```python
from build123d import *

# Parameters (mm, degrees)
SKETCH1_W           = 10
SKETCH1_H           = 12.5
SKETCH1_W_2         = 91
SKETCH1_H_2         = 10
SKETCH1_R           = 1.75
BOSS_EXTRUDE1_DEPTH = 3
SKETCH1_3_W         = 2
SKETCH1_3_H         = 10
SKETCH1_3_W_2       = 10
SKETCH1_3_H_2       = 2
BOSS_EXTRUDE2_DEPTH = 24
SKETCH2_W           = 10
SKETCH2_H           = 5
SKETCH2_W_2         = 5
SKETCH2_H_2         = 10
BOSS_EXTRUDE3_DEPTH = 2
SKETCH3_R           = 1.75
CUT_EXTRUDE1_DEPTH  = 12


with BuildPart() as part:
    # Sketch1 → Boss-Extrude1 (new body)
    # profile 1 of 5: a face of its own
    with BuildSketch(Plane(origin=(0, 0, 0), x_dir=(1, 0, 0), z_dir=(0, 1, 0))):
        with Locations((-10.142857143, 23.178571429)):
            Rectangle(SKETCH1_W, SKETCH1_H)
    # profile 2 of 5: a face of its own
    with BuildSketch(Plane(origin=(0, 0, 0), x_dir=(1, 0, 0), z_dir=(0, 1, 0))):
        with Locations((10.357142857, 11.928571429)):
            Rectangle(SKETCH1_W_2, SKETCH1_H_2)
        with Locations(Location((30.357142857, 11.928571429, 0), (0, 0, 270))):
            Circle(SKETCH1_R, mode=Mode.SUBTRACT)
        with Locations(Location((-9.642857143, 11.928571429, 0), (0, 0, 270))):
            Circle(SKETCH1_R, mode=Mode.SUBTRACT)
    # profile 3 of 5: a face of its own
    with BuildSketch(Plane(origin=(0, 0, 0), x_dir=(1, 0, 0), z_dir=(0, 1, 0))):
        with Locations((-10.142857143, 0.678571429)):
            Rectangle(SKETCH1_W, SKETCH1_H)
    # profile 4 of 5: a face of its own
    with BuildSketch(Plane(origin=(0, 0, 0), x_dir=(1, 0, 0), z_dir=(0, 1, 0))):
        with Locations((30.857142857, 0.678571429)):
            Rectangle(SKETCH1_W, SKETCH1_H)
    # profile 5 of 5: a face of its own
    with BuildSketch(Plane(origin=(0, 0, 0), x_dir=(1, 0, 0), z_dir=(0, 1, 0))):
        with Locations((30.857142857, 23.178571429)):
            Rectangle(SKETCH1_W, SKETCH1_H)
    extrude(amount=BOSS_EXTRUDE1_DEPTH)

    # Sketch1_3 → Boss-Extrude2 (add)
    with BuildSketch(Plane(origin=(0, 0, 0), x_dir=(1, 0, 0), z_dir=(0, 1, 0))):
        with Locations((-36.142857143, 11.928571429)):
            Rectangle(SKETCH1_3_W, SKETCH1_3_H)
        with Locations((-10.142857143, -6.571428571)):
            Rectangle(SKETCH1_3_W_2, SKETCH1_3_H_2)
        with Locations((30.857142857, -6.571428571)):
            Rectangle(SKETCH1_3_W_2, SKETCH1_3_H_2)
        with Locations((56.857142857, 11.928571429)):
            Rectangle(SKETCH1_3_W, SKETCH1_3_H)
        with Locations((30.857142857, 30.428571429)):
            Rectangle(SKETCH1_3_W_2, SKETCH1_3_H_2)
        with Locations((-10.142857143, 30.428571429)):
            Rectangle(SKETCH1_3_W_2, SKETCH1_3_H_2)
    extrude(amount=BOSS_EXTRUDE2_DEPTH)

    # Sketch2 → Boss-Extrude3 (add)
    with BuildSketch(Plane(origin=(0, 24, 0), x_dir=(1, 0, 0), z_dir=(0, 1, 0))):
        with Locations((-10.142857143, 28.928571429)):
            Rectangle(SKETCH2_W, SKETCH2_H)
        with Locations((30.857142857, 28.928571429)):
            Rectangle(SKETCH2_W, SKETCH2_H)
        with Locations((55.357142857, 11.928571429)):
            Rectangle(SKETCH2_W_2, SKETCH2_H_2)
        with Locations((30.857142857, -5.071428571)):
            Rectangle(SKETCH2_W, SKETCH2_H)
        with Locations((-10.142857143, -5.071428571)):
            Rectangle(SKETCH2_W, SKETCH2_H)
        with Locations((-34.642857143, 11.928571429)):
            Rectangle(SKETCH2_W_2, SKETCH2_H_2)
    extrude(amount=BOSS_EXTRUDE3_DEPTH)

    # Sketch3 → Cut-Extrude1 (cut)
    with BuildSketch(Plane.XZ):
        with Locations(Location((-10.142857143, -25.428571429, 0), (0, 0, 270))):
            Circle(SKETCH3_R)
        with Locations(Location((30.857142857, -25.428571429, 0), (0, 0, 270))):
            Circle(SKETCH3_R)
    extrude(amount=-CUT_EXTRUDE1_DEPTH, mode=Mode.SUBTRACT)


solid = part.part
```
Geometry: final body of the model. Coordinates: model frame, mm. A direction names the side the tool comes from. Round coordinates to 2 decimals unless told otherwise and drop trailing zeros. Order: outer loops, then holes, each group sorted by start corner. A loop starts at its lowest first (then second) coordinate and runs counter-clockwise, first axis right, second up. Notation, with made-up numbers: (19.25, 44.25) -> (34.25, 44.25) arc R37 ccw to (34.25, 80.25) -> close; hole circle Ø8 at (52, -36). An arc over 180 degrees is marked (long way). Use one line per item in the form item = value.
(1) Section D-D on z = -11.5. Return loops of the section in (x, y), and give its area (3 significant figures).
Results list:
outline = (-37.14, 0) -> (-11.34, 0) -> (-11.34, 3) -> (-35.14, 3) -> (-35.14, 24) -> (-32.14, 24) -> (-32.14, 26) -> (-37.14, 26) -> close; (-7.95, 0) -> (28.66, 0) -> (28.66, 3) -> (-7.95, 3) -> close; (32.05, 0) -> (57.86, 0) -> (57.86, 26) -> (52.86, 26) -> (52.86, 24) -> (55.86, 24) -> (55.86, 3) -> (32.05, 3) -> close
area = 369 mm^2
(2) Section B-B on z = 4. Return loops of the section in (x, y), and give its area (3 significant figures).
Results list:
outline = (-15.14, 0) -> (-5.14, 0) -> (-5.14, 3) -> (-15.14, 3) -> close; (-15.14, 24) -> (-5.14, 24) -> (-5.14, 26) -> (-15.14, 26) -> close; (25.86, 0) -> (35.86, 0) -> (35.86, 3) -> (25.86, 3) -> close; (25.86, 24) -> (35.86, 24) -> (35.86, 26) -> (25.86, 26) -> close
area = 100 mm^2
(3) Draft query along Y for faces 1 (the face through (-10, 13, -29.429)), 2 (the face through (-10, 26, 5)), 3 (the face through (31, 25, -26.429)). Return one class per face: pulls with the +Y half, pulls with the -Y half, needs draft (parallel to the pull), parting line crosses it, or undercut.
Results list:
face_1 = undercut
face_2 = pulls with the +Y half
face_3 = needs draft
(4) Section A-A on y = 8. Return loops of the section in (x, z), and give its area (3 significant figures).
Results list:
outline = (-37.14, -16.93) -> (-35.14, -16.93) -> (-35.14, -6.93) -> (-37.14, -6.93) -> close; (-15.14, -31.43) -> (-5.14, -31.43) -> (-5.14, -29.43) -> (-15.14, -29.43) -> close; (-15.14, 5.57) -> (-5.14, 5.57) -> (-5.14, 7.57) -> (-15.14, 7.57) -> close; (25.86, -31.43) -> (35.86, -31.43) -> (35.86, -29.43) -> (25.86, -29.43) -> close; (25.86, 5.57) -> (35.86, 5.57) -> (35.86, 7.57) -> (25.86, 7.57) -> close; (55.86, -16.93) -> (57.86, -16.93) -> (57.86, -6.93) -> (55.86, -6.93) -> close
area = 120 mm^2
(5) Section C-C on x = -7. Return loops of the section in (y, z).
Results list:
outline = (0, -31.43) -> (26, -31.43) -> (26, -26.43) -> (24, -26.43) -> (24, -29.43) -> (3, -29.43) -> (3, 5.57) -> (24, 5.57) -> (24, 2.57) -> (26, 2.57) -> (26, 7.57) -> (0, 7.57) -> close
(6) Ray query, probe 1 along X at (y, z) = (20.5, -16.5); probe 2 along X at (y, z) = (25, 4.5); probe 3 along Y at (x, z) = (53.5, -7). Return the intervals inside material, ascending. Write a range as [from, to].
Results list:
probe_1 = [-37.14, -35.14], [55.86, 57.86]
probe_2 = [-15.14, -5.14], [25.86, 35.86]
probe_3 = [0, 3], [24, 26]
(7) Access query for faces 4 (the face through (54, 24, -12)), 5 (the face through (31, 25, 2.571)), 6 (the face through (52.857, 25, -12)). Directions: +Z, -Z, +X, -X, +Y, -Y. A direction counts if a zero-diameter tool reaches every point of the face in a straight line with its end or side. Return the directions, or none.
Results list:
face_4 = +Z, -Z
face_5 = +X, -X, +Y
face_6 = +Z, -Z, +Y
(8) First-contact query: pin 1 Ø3 at (x, y) = (5.5, 2.5) entering from -Z; pin 2 Ø1.5 at (x, y) = (15, 1.5) entering from +Z; pin 3 Ø3 at (x, y) = (23.5, 23) entering from -Z; pin 4 Ø11.5 at (y, z) = (14.5, 1) entering from -X. Flat tips, straight axial feed; report the tip coordinate or a pass-through.
Results list:
pin_1 = -16.93
pin_2 = -6.93
pin_3 = through
pin_4 = -15.14
